Work out the finished part from the listing and answer in its coordinate system (mm). Round coordinates to 2 decimals unless told otherwise and drop trailing zeros. Order: outer loops, then holes, each group sorted by start corner. A loop starts at its lowest first (then second) coordinate and runs counter-clockwise, first axis right, second up. Notation, with made-up numbers: (65, -31.75) - (116, -31.75) arc R22 cw to (116, -12.75) - close; hole circle Ø7 at (0, 30). An arc over 180 degrees is marked (long way). Use CSV: the item, a comma, the result in double quotes.
from build123d import *

# Parameters (mm, degrees)
SKETCH1_R           = 19.5
SKETCH1_R_2         = 1.4
BOSS_EXTRUDE1_DEPTH = 6


with BuildPart() as part:
    # Sketch1 → Boss-Extrude1 (new body)
    with BuildSketch(Plane.XY):
        with Locations((8.397290399, 31.494734579)):
            Circle(SKETCH1_R)
        with Locations((8.397290399, 48.994734579)):
            Circle(SKETCH1_R_2, mode=Mode.SUBTRACT)
        with Locations((-9.102709601, 31.494734579)):
            Circle(SKETCH1_R_2, mode=Mode.SUBTRACT)
        with Locations((8.397290399, 13.994734579)):
            Circle(SKETCH1_R_2, mode=Mode.SUBTRACT)
        with Locations((25.897290399, 31.494734579)):
            Circle(SKETCH1_R_2, mode=Mode.SUBTRACT)
    extrude(amount=BOSS_EXTRUDE1_DEPTH)


solid = part.part
(1) Each of these flat-tipped pins is pushed along its axis until it touches: pin 1 (3 mm diameter, centred on y = 44.5, z = 3, fed in from -X); pin 2 (3 mm diameter, centred on y = 17, z = 5, fed in from -X). Where does it stop, or does it pass through?
Findings below:
pin 1,"stops at x = -7.35"
pin 2,"stops at x = -6.14"
(2) Find section C-C (y = 26.5). Determine the outline of the cut face in (x, z).
Findings below:
outline,"(-10.45, 0) - (27.25, 0) - (27.25, 6) - (-10.45, 6) - close"
(3) Find section B-B (x = -7). Determine the outline of the cut face in (y, z), and give its area (3 significant figures).
Findings below:
outline,"(19.53, 0) - (43.46, 0) - (43.46, 6) - (19.53, 6) - close"
area,"144 mm²"
(4) The mould has two halves that part along Y. Classify faces 1 (the cylindrical face through (18.88, 47.937, 2.958)), 2 (the cylindrical face through (7, 14.1, 3)), 3 (the flat face through (8, 32, 6)): released by +Y, released by -Y, zero draft, split by the parting line, or undercut.
Findings below:
face 1,"split by the parting line"
face 2,"undercut"
face 3,"zero draft"
(5) Find the intervals of material crossed by L1, parallel to X at y = 31, z = 2.95; L2, parallel to X at y = 42.5, z = 4.7; L3, parallel to Y at x = 25, z = 2.9, in increasing order. Write a range as from..to.
Findings below:
L1,"x = -11.1..-10.41, -7.79..24.59, 27.21..27.89"
L2,"x = -7.7..24.49"
L3,"y = 21.27..30.42, 32.57..41.72"
(6) Find section A-A (z = 2.2). Determine the outline of the cut face in (x, y).
Findings below:
outline,"circle Ø39 at (8.4, 31.49); hole circle Ø2.8 at (-9.1, 31.49); hole circle Ø2.8 at (8.4, 13.99); hole circle Ø2.8 at (8.4, 48.99); hole circle Ø2.8 at (25.9, 31.49)"
